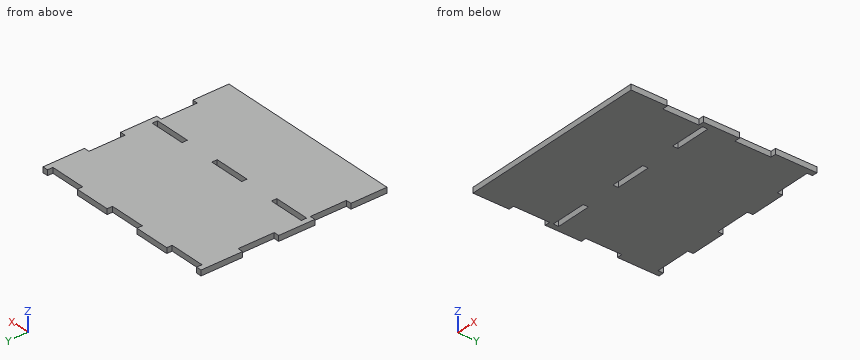
from build123d import *

# Parameters (mm, degrees)
SKETCH1_W           = 100
SKETCH1_H           = 100
BOSS_EXTRUDE1_DEPTH = 3
SKETCH2_W           = 20
SKETCH2_H           = 3
BOSS_EXTRUDE3_DEPTH = 3
SKETCH3_W           = 20
SKETCH3_H           = 3
BOSS_EXTRUDE4_DEPTH = 3
SKETCH5_W           = 3
SKETCH5_H           = 23
SKETCH5_H_2         = 20
BOSS_EXTRUDE5_DEPTH = 3
SKETCH6_W           = 3
SKETCH6_H           = 23
SKETCH6_H_2         = 20
BOSS_EXTRUDE6_DEPTH = 3
SKETCH7_W           = 20
SKETCH7_H           = 3
CUT_EXTRUDE1_DEPTH  = 3


with BuildPart() as part:
    # Sketch1 → Boss-Extrude1 (new body)
    with BuildSketch(Plane.XY):
        with Locations((50, 50)):
            Rectangle(SKETCH1_W, SKETCH1_H)
    extrude(amount=BOSS_EXTRUDE1_DEPTH)

    # Sketch2 → Boss-Extrude3 (add)
    with BuildSketch(Plane(origin=(0, 0, 0), x_dir=(-1, 0, 0), z_dir=(0, 0, -1))):
        with Locations((-30, 101.5)):
            Rectangle(SKETCH2_W, SKETCH2_H)
    extrude(amount=-BOSS_EXTRUDE3_DEPTH)

    # Sketch3 → Boss-Extrude4 (add)
    with BuildSketch(Plane.XY.offset(3)):
        with Locations((70, 101.5)):
            Rectangle(SKETCH3_W, SKETCH3_H)
    extrude(amount=-BOSS_EXTRUDE4_DEPTH)

    # Sketch5 → Boss-Extrude5 (add)
    with BuildSketch(Plane(origin=(0, 0, 0), x_dir=(-1, 0, 0), z_dir=(0, 0, -1))):
        with Locations((-101.5, 91.5)):
            Rectangle(SKETCH5_W, SKETCH5_H)
        with Locations((-101.5, 50)):
            Rectangle(SKETCH5_W, SKETCH5_H_2)
        with Locations((-101.5, 10)):
            Rectangle(SKETCH5_W, SKETCH5_H_2)
    extrude(amount=-BOSS_EXTRUDE5_DEPTH)

    # Sketch6 → Boss-Extrude6 (add)
    with BuildSketch(Plane(origin=(0, 0, 0), x_dir=(-1, 0, 0), z_dir=(0, 0, -1))):
        with Locations((1.5, 91.5)):
            Rectangle(SKETCH6_W, SKETCH6_H)
        with Locations((1.5, 50)):
            Rectangle(SKETCH6_W, SKETCH6_H_2)
        with Locations((1.5, 10)):
            Rectangle(SKETCH6_W, SKETCH6_H_2)
    extrude(amount=-BOSS_EXTRUDE6_DEPTH)

    # Sketch7 → Cut-Extrude1 (cut)
    with BuildSketch(Plane.XY.offset(3)):
        with Locations((10, 43.5)):
            Rectangle(SKETCH7_W, SKETCH7_H)
        with Locations((50, 43.5)):
            Rectangle(SKETCH7_W, SKETCH7_H)
        with Locations((90, 43.5)):
            Rectangle(SKETCH7_W, SKETCH7_H)
    extrude(amount=-CUT_EXTRUDE1_DEPTH, mode=Mode.SUBTRACT)


solid = part.part
Geometry: final body of the model. Coordinates: model frame, mm. Give positions to 0.01 mm unless a question says otherwise; leave off trailing zeros. Order: outer loops, then holes, each group sorted by start corner. A loop starts at its lowest first (then second) coordinate and runs counter-clockwise, first axis right, second up. Notation, with made-up numbers: (58, -37.75) -> (82, -37.75) arc R26 ccw to (82, -21.75) -> close; hole circle Ø3 at (9.25, 19). An arc over 180 degrees is marked (long way). Put each result on its own line as item: value.
Q1. Material intervals for L1, parallel to Y at x = 56, z = 2.75; L2, parallel to X at y = 32, z = 0.65, sorted ascending.
Here are the results:
L1: y = 0 to 42, 45 to 100
L2: x = 0 to 100
Q2. Section A-A, the plane x = 48. Return loops of the section in (y, z), then the cut area to 3 significant figures.
Here are the results:
outline: (0, 0) -> (42, 0) -> (42, 3) -> (0, 3) -> close; (45, 0) -> (100, 0) -> (100, 3) -> (45, 3) -> close
area: 291 mm^2
Q3. Section C-C, the plane y = 34. Return loops of the section in (x, z), then the cut area to 3 significant figures.
Here are the results:
outline: (0, 0) -> (100, 0) -> (100, 3) -> (0, 3) -> close
area: 300 mm^2
Q4. Pin query (flat end, axial travel): pin 1 (6 mm diameter, centred on x = 47.5, y = 77, fed in from -Z); pin 2 (0.9 mm diameter, centred on x = 45, z = 2, fed in from +Y); pin 3 (0.9 mm diameter, centred on y = 34.5, z = 2, fed in from +X). Return the tip coordinate at first contact, or that it passes through.
Here are the results:
pin 1: stops at z = 0
pin 2: stops at y = 100
pin 3: stops at x = 100
Q5. Section B-B, the plane z = 1.35. Count the separate pieces of the cut face and the enclosed holes in it, then the cut area to 3 significant figures.
Here are the results:
separate pieces: 1
enclosed holes: 3
area: 10,300 mm^2
